For this review, use the dimensioned drawing (mm, ordinates from the lowest corner) and the shaded views. A direction names the side the tool comes from. Coordinates: 2 decimals unless noted, no trailing zeros. Loops run counter-clockwise (first coordinate to the right, second up) from the corner with the lowest first, then second, coordinate; pieces in that order, holes last. Notation, with made-up numbers: (-32.75, 60.25) -> (-21.75, 60.25) arc R20 cw to (-21.75, 92.25) -> close; hole circle Ø3 at (-17, 44). An arc over 180 degrees is marked (long way). Answer as a JSON object with one key per item and string values.
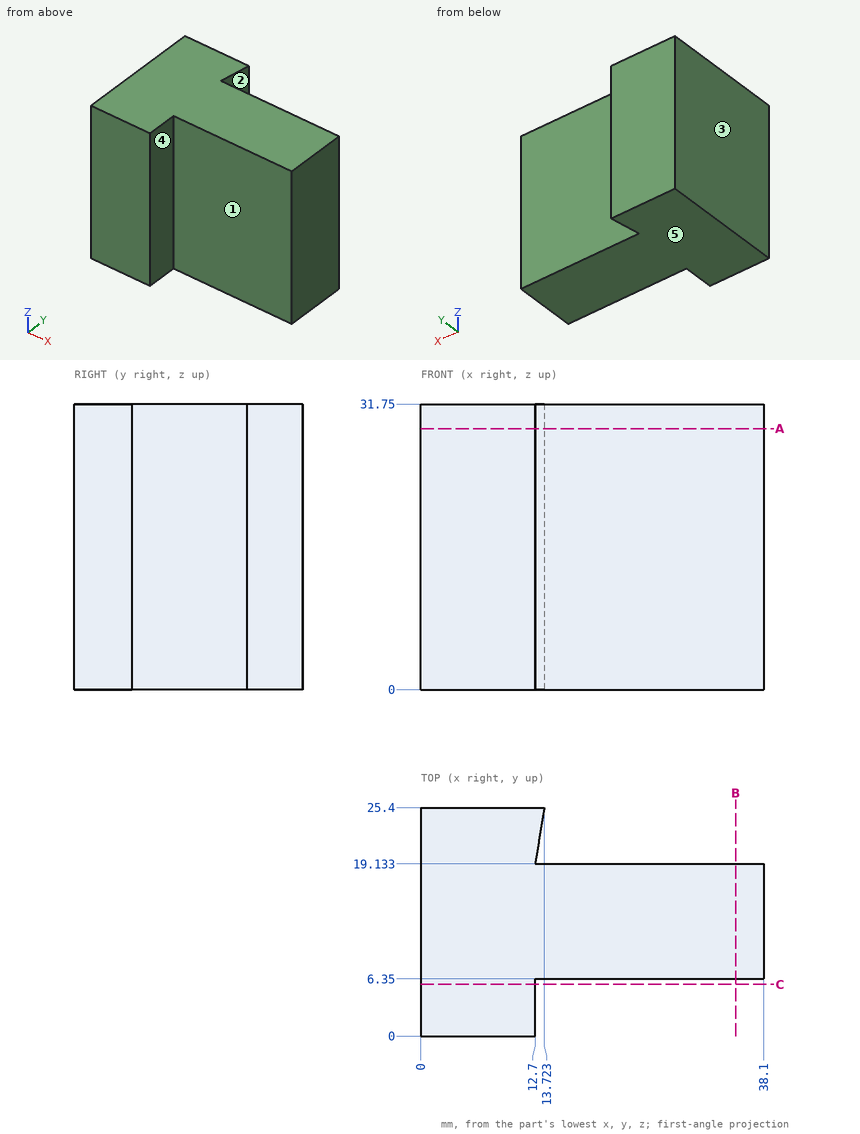
1) For the marked faces 4 and 5, list the 3-axis set-ups (+Z, -Z, +X, -X, +Y, -Y) from which the entire face can be reached by the end or side of a thin tool; tool diameter is ignored.
Completed:
{"face 4": "+Z, -Z, +X, -Y", "face 5": "-Z, +X, -X, +Y, -Y"}
2) Clearance check with flat-ended pins moving along their axes: pin 1 Ø12 at (x, z) = (32, 20) entering from +Y; pin 2 Ø5 at (y, z) = (2, 20) entering from +X. State where each tip first meets the part, or that it passes through.
Completed:
{"pin 1": "y = 19.13", "pin 2": "x = 12.7"}
3) The part is to be moulded in two halves that separate along Y. For the marked faces 1, 2 and 3, say which applies: pulls with the +Y half, pulls with the -Y half, needs draft (parallel to the pull), parting line crosses it, or undercut.
Completed:
{"face 1": "pulls with the -Y half", "face 2": "undercut", "face 3": "needs draft"}
4) Add section A-A, the plane z = 29. Give the boundary of the cut face in (x, y), and give its area (3 significant figures).
Completed:
{"outline": "(0, 0) -> (12.7, 0) -> (12.7, 6.35) -> (38.1, 6.35) -> (38.1, 19.13) -> (12.7, 19.13) -> (13.72, 25.4) -> (0, 25.4) -> close", "area": "650 mm²"}
5) Add section B-B, the plane x = 35. Give the boundary of the cut face in (y, z), and give its area (3 significant figures).
Completed:
{"outline": "(6.35, 0) -> (19.13, 0) -> (19.13, 31.75) -> (6.35, 31.75) -> close", "area": "406 mm²"}
6) Add section C-C, the plane y = 5.75. Give the boundary of the cut face in (x, z).
Completed:
{"outline": "(0, 0) -> (12.7, 0) -> (12.7, 31.75) -> (0, 31.75) -> close"}
7) Wall thickness on probe 1 along Y at (x, z) = (18, 5); probe 2 along X at (y, z) = (1.75, 18.5); probe 3 along X at (y, z) = (22.75, 9): over which ranges is each line inside the solid? List them lowest first.
Completed:
{"probe 1": "6.35 to 19.13", "probe 2": "0 to 12.7", "probe 3": "0 to 13.29"}
